```python
from build123d import *

# Parameters (mm, degrees)
PAD074_DEPTH    = 7
POCKET073_DEPTH = 5
PAD075_DEPTH    = 2
SKETCH187_R     = 1.5
POCKET074_DEPTH = 7
SKETCH189_W     = 1
SKETCH189_H     = 6
PAD076_DEPTH    = 1
SKETCH190_R     = 4.5
PAD077_DEPTH    = 1
SKETCH191_R     = 3.25
POCKET075_DEPTH = 4
SKETCH192_W     = 6
SKETCH192_H     = 1
POCKET076_DEPTH = 1


with BuildPart() as part:
    # Sketch184 → Pad074 (new body)
    with BuildSketch(Plane.XY):
        with BuildLine():
            ThreePointArc((-21.213203, 21.213203), (0, -30), (21.213203, 21.213203))
            Line((25.455844, 25.455844), (21.213203, 21.213203))
            ThreePointArc((-25.455844, 25.455844), (0, -36), (25.455844, 25.455844))
            Line((-25.455844, 25.455844), (-21.213203, 21.213203))
        make_face()
    extrude(amount=PAD074_DEPTH)

    # Sketch185 (on Face6 of Pad074) → Pocket073 (cut)
    with BuildSketch(Plane.XY.offset(7)):
        with BuildLine():
            ThreePointArc((-23.79351, 21.397871), (0, -32), (23.79351, 21.397871))
            Line((25.164596, 22.863577), (23.79351, 21.397871))
            ThreePointArc((-25.164596, 22.863577), (0, -34), (25.164596, 22.863577))
            Line((-25.164596, 22.863577), (-23.79351, 21.397871))
        make_face()
    extrude(amount=-POCKET073_DEPTH, mode=Mode.SUBTRACT)

    # Sketch186 (on Face5 of Pocket073) → Pad075 (join)
    with BuildSketch(Plane.XY.offset(7)):
        with BuildLine():
            ThreePointArc((-21.213203, 21.213203), (0, -30), (21.213203, 21.213203))
            Line((25.455844, 25.455844), (21.213203, 21.213203))
            ThreePointArc((-25.455844, 25.455844), (0, -36), (25.455844, 25.455844))
            Line((-25.455844, 25.455844), (-21.213203, 21.213203))
        make_face()
    extrude(amount=PAD075_DEPTH)

    # Sketch187 (on Face10 of Pad075) → Pocket074 (cut)
    with BuildSketch(Plane.XY.offset(9)):
        with Locations((-25.677783, 20.728036)):
            Circle(SKETCH187_R)
        with Locations((-30.707527, 12.085023)):
            Circle(SKETCH187_R)
        with Locations((-32.91748, 2.332274)):
            Circle(SKETCH187_R)
        with Locations((-32.104708, -7.634641)):
            Circle(SKETCH187_R)
        with Locations((-28.343844, -16.900488)):
            Circle(SKETCH187_R)
        with Locations((-21.980241, -24.614407)):
            Circle(SKETCH187_R)
        with Locations((-13.598249, -30.06805)):
            Circle(SKETCH187_R)
        with Locations((-3.967567, -32.760623)):
            Circle(SKETCH187_R)
        with Locations((3.967567, -32.760623)):
            Circle(SKETCH187_R)
        with Locations((13.598249, -30.06805)):
            Circle(SKETCH187_R)
        with Locations((21.980241, -24.614407)):
            Circle(SKETCH187_R)
        with Locations((28.343844, -16.900488)):
            Circle(SKETCH187_R)
        with Locations((32.104708, -7.634641)):
            Circle(SKETCH187_R)
        with Locations((32.91748, 2.332274)):
            Circle(SKETCH187_R)
        with Locations((30.707527, 12.085023)):
            Circle(SKETCH187_R)
        with Locations((25.677783, 20.728036)):
            Circle(SKETCH187_R)
    extrude(amount=-POCKET074_DEPTH, mode=Mode.SUBTRACT)

    # Sketch189 (on Face1 of Pocket074) → Pad076 (join)
    with BuildSketch(Plane(origin=(0, 0, 0), x_dir=(1, 0, 0), z_dir=(0, 0, -1))):
        with Locations((0.5, 33)):
            Rectangle(SKETCH189_W, SKETCH189_H)
    extrude(amount=PAD076_DEPTH)

    # Sketch190 (on Face14 of Pad076) → Pad077 (join)
    with BuildSketch(Plane.XZ.offset(36)):
        with Locations((0, 4.5)):
            Circle(SKETCH190_R)
    extrude(amount=-PAD077_DEPTH)

    # Sketch191 (on Face13 of Pad077) → Pocket075 (cut)
    with BuildSketch(Plane.XZ.offset(36)):
        with Locations((0, 4.5)):
            Circle(SKETCH191_R)
    extrude(amount=-POCKET075_DEPTH, mode=Mode.SUBTRACT)

    # Sketch192 (on Face35 of Pocket075) → Pocket076 (cut)
    with BuildSketch(Plane.YZ.offset(1)):
        with Locations((-33, -0.5)):
            Rectangle(SKETCH192_W, SKETCH192_H)
    extrude(amount=-POCKET076_DEPTH, mode=Mode.SUBTRACT)


solid = part.part
```
Geometry: final body of the model. Coordinates: model frame, mm. A direction names the side the tool comes from. Round coordinates to 2 decimals unless told otherwise and drop trailing zeros. Order: outer loops, then holes, each group sorted by start corner. A loop starts at its lowest first (then second) coordinate and runs counter-clockwise, first axis right, second up. Notation, with made-up numbers: (83, 77.5) -> (118, 77.5) arc R9 ccw to (118, 84.5) -> close; hole circle Ø9 at (71.25, 32.5). An arc over 180 degrees is marked (long way). Use CSV: the item, a comma, the result in double quotes. Start each with the question number.
1) Section C-C (y = -27). Return the cut outline in (x, z), and give its area (3 significant figures).
2) First-contact query: pin 1 Ø4 at (y, z) = (9, 3) entering from -X; pin 2 Ø2.5 at (x, y) = (-32.1, -7.63) entering from +Z; pin 3 Ø1.5 at (y, z) = (13, 6.5) entering from +X. Flat tips, straight axial feed; report the tip coordinate or a pass-through.
3) Set-up query: faces 1 (the face through (20.875, -23.601, 6.327)), 2 (the face through (-29.67, -11.99, 4.54)). Return all of +Z, -Z, +X, -X, +Y, -Y with unobstructed straight access to the full face (end or side cutting, diameter ignored); none if empty.
4) Section A-A (y = 0). Return the cut outline in (x, z).
5) Material intervals for line 1 along X through (y, z) = (0, 6); line 2 along X through (y, z) = (2, 3.5); line 3 along Z through (x, y) = (27.5, 17.5), sorted ascending. Write a range as from..to.
6) Draft query along Y for faces 3 (the face through (23, 23, 4)), 4 (the face through (33.17, 7.46, 4.54)). Return one class per face: +Y half, -Y half, draft (parallel to the pull), parting line (faces both ways), or undercut.
7) Section B-B (x = -9). Return the cut outline in (y, z).
Returned:
1,outline,"(-23.81, 0) -> (-13.08, 0) -> (-13.08, 9) -> (-23.81, 9) -> close; (13.08, 0) -> (23.81, 0) -> (23.81, 9) -> (13.08, 9) -> close; hole (-20.66, 2) -> (-17.18, 2) -> (-17.18, 7) -> (-20.66, 7) -> close; hole (17.18, 2) -> (20.66, 2) -> (20.66, 7) -> (17.18, 7) -> close"
1,area,"158 mm²"
2,pin 1,"stops at x = -35.31"
2,pin 2,"stops at z = 2"
2,pin 3,"stops at x = 33.85"
3,face 1,"+Z"
3,face 2,"none"
4,outline,"(-36, 0) -> (-30, 0) -> (-30, 9) -> (-36, 9) -> close; (30, 0) -> (36, 0) -> (36, 9) -> (30, 9) -> close; hole (-34, 2) -> (-32, 2) -> (-32, 7) -> (-34, 7) -> close; hole (32, 2) -> (34, 2) -> (34, 7) -> (32, 7) -> close"
5,line 1,"x = -36..-34, -32..-30, 30..32, 34..36"
5,line 2,"x = -35.94..-34.38, -31.45..-29.93, 29.93..31.45, 34.38..35.94"
5,line 3,"z = 0..2, 7..9"
6,face 3,"+Y half"
6,face 4,"undercut"
7,outline,"(-34.86, 0) -> (-28.62, 0) -> (-28.62, 9) -> (-34.86, 9) -> close; hole (-32.79, 2) -> (-30.71, 2) -> (-30.71, 7) -> (-32.79, 7) -> close"
